For this review, take the finished solid that the model builds, in its own axes (mm). A direction names the side the tool comes from. Give positions to 0.01 mm unless a question says otherwise; leave off trailing zeros. Write each loop counter-clockwise with the first axis right and the second up, starting at its lowest first coordinate (ties: lowest second). Pieces come first, ordered by that corner, then holes. Notation, with made-up numbers: (84.25, -39) -> (127.25, -39) arc R12 ccw to (127.25, -21) -> close; hole circle Ø11 at (51, 81.5). An arc over 180 degrees is marked (long way). Return JSON: item names as keys, results as strings.
from build123d import *

# Parameters (mm, degrees)
SKETCH1_W           = 20
SKETCH1_H           = 15
BOSS_EXTRUDE1_DEPTH = 35
SKETCH2_R           = 4
CUT_EXTRUDE1_DEPTH  = 36
CHAMFER1_SIZE       = 2
CHAMFER2_SIZE       = 2
CHAMFER2_SIZE2      = 3.464101615
SKETCH4_W           = 2
SKETCH4_H           = 1
CUT_EXTRUDE2_DEPTH  = 16
SKETCH5_W           = 4
SKETCH5_H           = 8
SKETCH5_R           = 1.25
CUT_EXTRUDE3_DEPTH  = 1
SKETCH3_W           = 37.5
SKETCH3_H           = 6
BOSS_EXTRUDE2_DEPTH = 5
SKETCH6_W           = 8
SKETCH6_H           = 6
BOSS_EXTRUDE3_DEPTH = 2


with BuildPart() as part:
    # Sketch1 → Boss-Extrude1 (new body)
    with BuildSketch(Plane.XY):
        Rectangle(SKETCH1_W, SKETCH1_H)
    extrude(amount=BOSS_EXTRUDE1_DEPTH)

    # Sketch2 → Cut-Extrude1 (cut, through all)
    with BuildSketch(Plane.XY.offset(35)):
        Circle(SKETCH2_R)
    extrude(amount=-CUT_EXTRUDE1_DEPTH, mode=Mode.SUBTRACT)

    # Chamfer1
    chamfer1_edges = [part.edges().sort_by_distance(p)[0] for p in [
        (10, 7.5, 17.5),
        (10, -7.5, 17.5),
        (-10, -7.5, 17.5),
        (-10, 7.5, 17.5),
    ]]
    chamfer(chamfer1_edges, length=CHAMFER1_SIZE)

    # Chamfer2
    chamfer2_edges = [part.edges().sort_by_distance(p)[0] for p in [
        (-10, 0, 0),
        (0, 7.5, 0),
        (10, 0, 0),
        (0, -7.5, 0),
        (9, 6.5, 0),
        (9, -6.5, 0),
        (-9, -6.5, 0),
        (-9, 6.5, 0),
    ]]
    chamfer2_side = [part.faces().sort_by_distance(p)[0] for p in [
        (-9.75, 0, 0),
    ]]
    chamfer(chamfer2_edges, length=CHAMFER2_SIZE, length2=CHAMFER2_SIZE2, reference=chamfer2_side[0])

    # Sketch4 → Cut-Extrude2 (cut, through all)
    with BuildSketch(Plane.XZ.offset(7.5)):
        with Locations((-9, 11.732050808)):
            Rectangle(SKETCH4_W, SKETCH4_H)
        with Locations((-9, 13.482050808)):
            Rectangle(SKETCH4_W, SKETCH4_H)
        with Locations((-9, 15.232050808)):
            Rectangle(SKETCH4_W, SKETCH4_H)
        with Locations((-9, 16.982050808)):
            Rectangle(SKETCH4_W, SKETCH4_H)
        with Locations((-9, 18.732050808)):
            Rectangle(SKETCH4_W, SKETCH4_H)
        with Locations((9, 18.732050808)):
            Rectangle(SKETCH4_W, SKETCH4_H)
        with Locations((9, 16.982050808)):
            Rectangle(SKETCH4_W, SKETCH4_H)
        with Locations((9, 15.232050808)):
            Rectangle(SKETCH4_W, SKETCH4_H)
        with Locations((9, 13.482050808)):
            Rectangle(SKETCH4_W, SKETCH4_H)
        with Locations((9, 11.732050808)):
            Rectangle(SKETCH4_W, SKETCH4_H)
    extrude(amount=-CUT_EXTRUDE2_DEPTH, mode=Mode.SUBTRACT)

    # Sketch5 → Cut-Extrude3 (cut)
    with BuildSketch(Plane.XZ.offset(7.5)):
        with Locations((0, 10)):
            Rectangle(SKETCH5_W, SKETCH5_H)
        with Locations((0, 9)):
            Circle(SKETCH5_R, mode=Mode.SUBTRACT)
    extrude(amount=-CUT_EXTRUDE3_DEPTH, mode=Mode.SUBTRACT)

    # Sketch3 → Boss-Extrude2 (add)
    with BuildSketch(Plane(origin=(10, 0, 0), x_dir=(0, 0, -1), z_dir=(1, 0, 0))):
        with Locations((-28.75, 0)):
            Rectangle(SKETCH3_W, SKETCH3_H)
    extrude(amount=BOSS_EXTRUDE2_DEPTH)

    # Sketch6 → Boss-Extrude3 (add)
    with BuildSketch(Plane.ZY.offset(-10)):
        with Locations((15.232050808, 0)):
            Rectangle(SKETCH6_W, SKETCH6_H)
    extrude(amount=BOSS_EXTRUDE3_DEPTH)


solid = part.part
1. To check wall thickness, follow probe 1 along Y at (x, z) = (0, 15); probe 2 along Z at (x, y) = (9.5, 4.5); probe 3 along Z at (x, y) = (11, -0.25). State the ranges of each line that lie inside material, in increasing order.
Results found:
{"probe 1": "y = -7.5 to -4, 4 to 7.5", "probe 2": "z = 2.6 to 11.23, 12.23 to 12.98, 13.98 to 14.73, 15.73 to 16.48, 17.48 to 18.23, 19.23 to 35", "probe 3": "z = 10 to 47.5"}
2. Add section D-D, the plane z = 21.5. State the section outline as (x, y) points, plus the area to 3 significant figures.
Results found:
{"outline": "(-10, -5.5) -> (-8, -7.5) -> (8, -7.5) -> (10, -5.5) -> (10, -3) -> (15, -3) -> (15, 3) -> (10, 3) -> (10, 5.5) -> (8, 7.5) -> (-8, 7.5) -> (-10, 5.5) -> close; hole circle Ø8 at (0, 0)", "area": "272 mm²"}
3. For faces 1 (the flat face through (-8, 0, 15)), 2 (the flat face through (8, 5, 12)), 3 (the flat face through (9, -5, 12.232)), list the 3-axis set-ups (+Z, -Z, +X, -X, +Y, -Y) from which the entire face can be reached by the end or side of a thin tool; tool diameter is ignored.
Results found:
{"face 1": "-X, +Y, -Y", "face 2": "+X, +Y", "face 3": "+X, -Y"}
4. Add section A-A, the plane x = 0. State the section outline as (y, z) points, plus the area to 3 significant figures.
Results found:
{"outline": "(-7.5, 3.46) -> (-5.5, 0) -> (-4, 0) -> (-4, 35) -> (-7.5, 35) -> (-7.5, 14) -> (-6.5, 14) -> (-6.5, 10.25) -> (-7.5, 10.25) -> (-7.5, 7.75) -> (-6.5, 7.75) -> (-6.5, 6) -> (-7.5, 6) -> close; (4, 0) -> (5.5, 0) -> (7.5, 3.46) -> (7.5, 35) -> (4, 35) -> close", "area": "233 mm²"}
5. Add section B-B, the plane z = 9. State the section outline as (x, y) points, plus the area to 3 significant figures.
Results found:
{"outline": "(-10, -5.5) -> (-8, -7.5) -> (-2, -7.5) -> (-2, -6.5) -> (-1.25, -6.5) -> (-1.25, -7.5) -> (1.25, -7.5) -> (1.25, -6.5) -> (2, -6.5) -> (2, -7.5) -> (8, -7.5) -> (10, -5.5) -> (10, 5.5) -> (8, 7.5) -> (-8, 7.5) -> (-10, 5.5) -> close; hole circle Ø8 at (0, 0)", "area": "240 mm²"}
6. For pin 1 (0.8 mm diameter, centred on x = -0.5, y = -7, fed in from -Z); pin 2 (1.6 mm diameter, centred on x = 9.5, y = 5, fed in from +Z); pin 3 (2 mm diameter, centred on x = 12, y = -5.5, fed in from -Z); pin 4 (1.5 mm diameter, centred on x = 13.5, y = -0.5, fed in from -Z), all flat-tipped, find the tip position at first contact; note any pin that passes through.
Results found:
{"pin 1": "stops at z = 1.91", "pin 2": "stops at z = 35", "pin 3": "passes through", "pin 4": "stops at z = 10"}
